For this review, take the finished solid that the model builds, in its own axes (mm). Face numbers are marked on the shaded views. Coordinates: 2 decimals unless noted, no trailing zeros. Order: outer loops, then holes, each group sorted by start corner. A loop starts at its lowest first (then second) coordinate and runs counter-clockwise, first axis right, second up. Notation, with made-up numbers: (16.5, 41) - (40.5, 41) arc R17 cw to (40.5, 55) - close; hole circle Ø3 at (-8.5, -4.5). An arc over 180 degrees is marked (long way). One line per item, written item: value. Start each with the question number.
(1) To check wall thickness, follow line 1 along Z through (x, y) = (-1.6, -0.55); line 2 along X through (y, z) = (-0.1, -1.5); line 3 along X through (y, z) = (-0.95, -8). State the ranges of each line that lie inside material, in increasing order.
(2) Clearance check with flat-ended pins moving along their axes: pin 1 (0.8 mm diameter, centred on x = 0.5, z = 1.5, fed in from -Y); pin 2 (1.1 mm diameter, centred on x = 0, z = 1.5, fed in from +Y); pin 3 (3 mm diameter, centred on x = -2, z = -6, fed in from +Y). State where each tip first meets the part, or that it passes through.
(3) Consider section A-A on z = -5. Write out the cut boundary in (x, y), then the cut area to 3 significant figures.
(4) Mouldability with a two-part tool opening along Y and no side actions: class the marked faces 1, 2, 3 and 4 as released by +Y, released by -Y, zero draft, split by the parting line, or undercut.
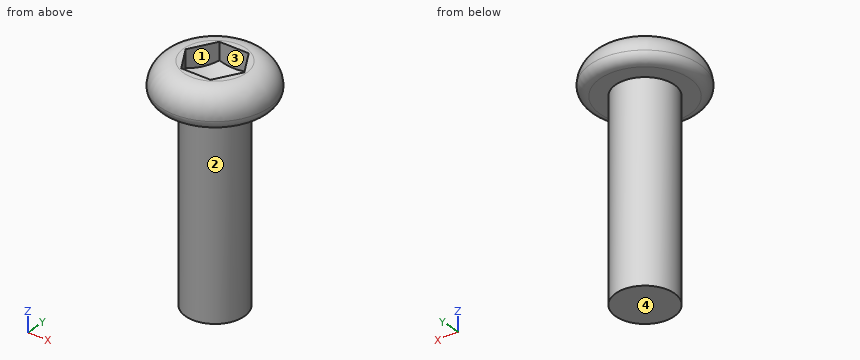
Autodesk Inventor part; units mm, degrees
ref_plane "YZ Plane" through (0, 0, 0) normal (1, 0, 0) x (0, 1, 0)
ref_plane "XZ Plane" through (0, 0, 0) normal (0, 1, 0) x (-1, 0, 0)
ref_plane "XY Plane" through (0, 0, 0) normal (0, 0, 1) x (1, 0, 0)
sketch "Sketch1" plane through (0, 0, 0) normal (0, 0, 1) x (1, 0, 0)
  circle A0 centre (0, 0) radius 2.8
  dimension "d0" = 5.6
extrude "Extrusion1" add sketch "Sketch1" along normal blind 1.7
fillet "Fillet3" radius 0.5 1 edges at (-2.8, 0, 0)
fillet "Fillet4" radius 1.2 1 edges at (-2.8, 0, 1.7)
sketch "Sketch2" plane through (0, 0, 1.7) normal (0, 0, 1) x (1, 0, 0)
  line L0 (-0.75, -1.299) -> (0.75, -1.299)
  line L1 (0.75, -1.299) -> (1.5, 0)
  line L2 (1.5, 0) -> (0.75, 1.299)
  line L3 (0.75, 1.299) -> (-0.75, 1.299)
  line L4 (-0.75, 1.299) -> (-1.5, 0)
  line L5 (-1.5, 0) -> (-0.75, -1.299)
  dimension "d7" = 3
extrude "Extrusion2" cut sketch "Sketch2" against normal blind 1.7
sketch "Sketch3" plane through (0, 0, 0) normal (0, 1, 0) x (-1, 0, 0)
  line L0 (0, 0) -> (1.5, 0)
  line L1 (2.3, 0) -> (-2.3, 0)
  line L2 (1.5, 0) -> (1.5, 0.8)
  line L3 (1.5, 0.8) -> (0, 0)
  line L4 (0, 0) -> (0, 2.432)
  dimension "d13" = 0
  dimension "d14" = 1.5
  dimension "d15" = 0.8
revolve "Revolution2" add sketch "Sketch3" angle 360 about axis through (0, 0, 0) along (0, 0, 1)
sketch "Sketch4" plane through (0, 0, 0) normal (0, 0, -1) x (-1, 0, 0)
  circle A0 centre (0, 0) radius 2.3
  circle A1 centre (0, 0) radius 1.5
  dimension "d18" = 3
extrude "Extrusion3" add sketch "Sketch4" along normal blind 10 contours A1
thread "Thread1"
properties part number "screw_M3_10_hex"
Geometry check:
1. line 1: z = 0 to 1.7
1. line 2: x = -1.5 to 1.5
1. line 3: x = -1.16 to 1.16
2. pin 1: stops at y = -2.6
2. pin 2: stops at y = 2.71
2. pin 3: stops at y = 1.41
3. outline: circle Ø3 at (0, 0)
3. area: 7.07 mm^2
4. face 1: undercut
4. face 2: split by the parting line
4. face 3: undercut
4. face 4: zero draft
